Autodesk Inventor part; units mm, degrees
ref_plane "YZ Plane" through (0, 0, 0) normal (1, 0, 0) x (0, 1, 0)
ref_plane "XZ Plane" through (0, 0, 0) normal (0, 1, 0) x (-1, 0, 0)
ref_plane "XY Plane" through (0, 0, 0) normal (0, 0, 1) x (1, 0, 0)
sketch "Sketch1" plane through (0, 0, 0) normal (0, 1, 0) x (-1, 0, 0)
  line L0 (-55.3, 34) -> (55.3, -34) construction
  line L1 (55.3424, 32) -> (55.3424, 21)
  line L2 (53.3, 10) -> (55.3, 10)
  line L3 (55.3, 10) -> (55.3, -1)
  line L4 (55.3, -1) -> (53.3, -1)
  line L5 (53.3, -1) -> (53.3, -12)
  line L6 (53.3, -12) -> (55.3, -12)
  line L7 (55.3, -12) -> (55.3, -23)
  line L8 (55.3, -23) -> (53.3, -23)
  line L9 (55.3424, 21) -> (55.3424, 32)
  line L10 (55.3, -23) -> (55.3, -12)
  line L11 (55.3, -1) -> (55.3, 10)
  line L12 (-53.3, 0.4465) -> (-53.3, 0.446)
  line L13 (-53.3487, -21) -> (-53.3, -21)
  line L14 (55.3424, 32) -> (37.0424, 32)
  line L15 (37.0424, 32) -> (37.0424, 34)
  line L16 (37.0424, 34) -> (18.7424, 34)
  line L17 (18.7424, 34) -> (18.7424, 32)
  line L18 (18.7424, 32) -> (-1.6, 32)
  line L19 (-1.6, 32) -> (-1.6, 34)
  line L20 (-1.6, 34) -> (-17.9, 34)
  line L21 (-17.9, 34) -> (-17.9, 32)
  line L22 (-17.9, 32) -> (-36.2, 32)
  line L23 (-36.2, 32) -> (-36.2, 34)
  line L24 (37.0424, 34) -> (18.7424, 34)
  line L25 (-1.6, 34) -> (-17.9, 34)
  line L26 (-36.2, 34) -> (-55.3, 34)
  line L27 (2.5632, 10.7554) -> (14.3549, 2.3144)
  line L28 (0.7434, 10.7554) -> (-11.0739, 2.3144)
  line L29 (19.1722, 2.3144) -> (2.5632, 14.178)
  line L30 (0.7434, 14.1963) -> (-15.8912, 2.3144)
  line L31 (-20.6639, 0.446) -> (0.7434, -14.8449)
  line L32 (2.5632, -14.8267) -> (23.9449, 0.446)
  line L33 (23.9895, 2.3144) -> (2.5632, 17.6189)
  line L34 (0.7434, 17.6372) -> (-20.7085, 2.3144)
  line L35 (-25.4812, 0.446) -> (0.7434, -18.2859)
  line L36 (2.5632, -18.2676) -> (28.7623, 0.446)
  line L37 (28.8068, 2.3144) -> (2.5632, 21.0599)
  line L38 (41.2856, 32.5499) -> (41.2856, 32.5817)
  line L39 (54.8971, 24.1408) -> (54.9227, 24.1408)
  line L40 (14.3549, 0.446) -> (14.3549, 0.4779)
  line L41 (0.7434, 21.0782) -> (-25.5258, 2.3144)
  line L42 (-11.0739, 2.3144) -> (-15.8912, 2.3144)
  line L43 (-20.7085, 2.3144) -> (-25.5258, 2.3144)
  line L44 (0.7434, 21.0782) -> (0.7434, 17.6372)
  line L45 (0.7434, 14.1963) -> (0.7434, 10.7554)
  line L46 (2.5632, 10.7554) -> (2.5632, 14.178)
  line L47 (2.5632, 17.6189) -> (2.5632, 21.0599)
  line L48 (14.3549, 2.3144) -> (19.1722, 2.3144)
  line L49 (23.9895, 2.3144) -> (28.8068, 2.3144)
  line L50 (28.7623, 0.446) -> (23.9449, 0.446)
  line L51 (2.5632, -14.8267) -> (2.5632, -18.2676)
  line L52 (0.7434, -18.2859) -> (0.7434, -14.8449)
  line L53 (-25.4812, 0.446) -> (-20.6639, 0.446)
  line L54 (-11.0739, 0.4464) -> (-15.8912, 0.4464)
  line L55 (0.7434, -7.9945) -> (-11.0739, 0.4464)
  line L56 (0.7434, -11.4354) -> (-15.8912, 0.4464)
  line L57 (0.7434, -11.4354) -> (0.7434, -7.9945)
  line L58 (-11.7935, 1.3804) -> (-5.9618, 1.3804)
  line L59 (2.5632, 10.7554) -> (2.5632, 10.7554)
  line L60 (2.5632, -7.9945) -> (2.5632, -11.4171)
  line L61 (14.3549, 0.4464) -> (19.1722, 0.4464)
  line L62 (19.1722, 0.4464) -> (2.5632, -11.4171)
  line L63 (2.5632, -7.9945) -> (14.3549, 0.4464)
  line L64 (19.1722, 0.4464) -> (14.3549, 0.4464)
  line L65 (14.3549, 0.4464) -> (2.5632, -7.9945)
  line L66 (2.5632, -7.9945) -> (2.5632, -11.4171)
  line L67 (2.5632, -11.4171) -> (19.1722, 0.4464)
  line L68 (53.3, 10) -> (53.3, 21)
  line L69 (53.3, 21) -> (55.3424, 21)
  line L70 (53.3, -34.0004) -> (53.3, -34.0004)
  line L71 (53.3, -23) -> (53.3, -32)
  line L72 (34.2, -32.0004) -> (34.2, -32)
  line L73 (55.3, 34) -> (-52.0471, -32) construction
  line L74 (53.3, -32) -> (53.3, -34.0004)
  line L75 (-39, -36.0004) -> (-53.3, -36.0004)
  line L76 (-53.3, -36.0004) -> (-57.3, -36.0004)
  line L77 (-57.3, -36.0004) -> (-57.3, -21.0004)
  line L78 (-57.3, -21.0004) -> (-59.3, -21.0004)
  line L79 (-59.3, -21.0004) -> (-59.3, -9.7058)
  line L80 (-59.3, -9.7058) -> (-57.3, -9.7058)
  line L81 (-57.3, -9.7058) -> (-57.3, 0.4464)
  line L82 (-57.3, 0.4464) -> (-57.3, 1)
  line L83 (-57.3, 1) -> (-59.3, 1)
  line L84 (-59.3, 1) -> (-59.3, 12)
  line L85 (-59.3, 12) -> (-57.3, 12)
  line L86 (-57.3, 12) -> (-57.3, 23)
  line L87 (-57.3, 23) -> (-59.3, 23)
  line L88 (-59.3, 23) -> (-59.3, 34)
  line L89 (-59.3, 34) -> (-55.3, 34)
  line L90 (-53.3, -21) -> (-53.3, -21.0004)
  line L91 (-55.3, 32.0365) -> (-55.3, 32)
  line L92 (-55.3, 32.0365) -> (-55.3, 32)
  line L93 (-39, -36.0004) -> (-38.1942, -36.0004)
  line L94 (53.3, -34.0004) -> (35, -34.0004)
  line L95 (35, -34.0004) -> (35, -36.0004)
  line L96 (35, -36.0004) -> (18.7, -36.0004)
  line L97 (18.7, -36.0004) -> (16.7, -36.0004)
  line L98 (16.7, -36.0004) -> (16.7, -34.0004)
  line L99 (16.7, -34.0004) -> (-1.6, -34.0004)
  line L100 (-1.6, -34.0004) -> (-1.6, -36.0004)
  line L101 (-1.6, -36.0004) -> (-17.9, -36.0004)
  line L102 (-17.9, -36.0004) -> (-19.9, -36.0004)
  line L103 (-19.9, -36.0004) -> (-19.9, -34.0004)
  line L104 (-19.9, -34.0004) -> (-38.2, -34.0004)
  line L105 (-38.2, -34.0004) -> (-38.1942, -36.0004)
  point P0 (0, 0)
  point P1 (-53.3, 20.3166)
  point P2 (-53.3, 1)
  point P3 (-53.3, -10)
  point P4 (-55.3, -18.9529)
  point P5 (-53.3, -32.7703)
  point P6 (-16.7, -32.027)
  point P7 (-21.4801, -32.0004)
  point P8 (-17.9, -36.0004)
  dimension "d30" = 1.868
  dimension "d31" = 0.934
  dimension "d34" = 11
  dimension "d35" = 11
  dimension "d36" = 11
  dimension "d37" = 11
  dimension "d38" = 11
  dimension "d61" = 4
  dimension "d70" = 18.3
  dimension "d72" = 2
  dimension "d73" = 18.3
  dimension "d75" = 2
extrude "Extrusion1" add sketch "Sketch1" along normal blind 2
properties part number "ATAS"
Part model, mm, in its own coordinate system. A direction names the side the tool comes from. Round coordinates to 2 decimals unless told otherwise and drop trailing zeros. Loops run counter-clockwise (first coordinate to the right, second up) from the corner with the lowest first, then second, coordinate; pieces in that order, holes last. Notation, with made-up numbers: (79, -37) -> (111, -37) arc R7 ccw to (111, -31) -> close; hole circle Ø11 at (-32.75, -32.75). An arc over 180 degrees is marked (long way). Use one line per item in the form item = value. Start each with the question number.
Item 1: Band-saw the part on C-C (z = -5.5). List the corners of the cut face in (x, y), plus the area to 3 significant figures.
Item 2: Band-saw the part on D-D (y = 1.5). Give the number of separate pieces and of enclosed holes in the cut face, plus the area to 3 significant figures.
Item 3: Tool access for faces 1 (the flat face through (3, 0, -1)), 2 (the flat face through (12.207, 0.986, 11.828)): list every direction of +Z, -Z, +X, -X, +Y, -Y with a clear straight run to the whole face (end or side of a thin tool).
Item 4: Drop flat-ended pins along their axis: pin 1 Ø0.6 at (y, z) = (1.5, 20) entering from +X; pin 2 Ø1 at (x, y) = (-6.5, 1) entering from -Z; pin 3 Ø1 at (x, y) = (18.5, 1) entering from +Z. Give the stop position or say it passes through.
Item 5: Drill centre lines: line 1 along Z through (x, y) = (-8, 0.45); line 2 along X through (y, z) = (1.9, -1.5); line 3 along Z through (x, y) = (14.5, 0.35). Where is each one in solid material? Low to high.
Item 6: Band-saw the part on A-A (z = -13.5). List the corners of the cut face in (x, y).
Item 7: Band-saw the part on B-B (x = -21). List the corners of the cut face in (y, z).
Item 8: Two-plate mould, pull along Z, no slides. Class faces 3 (the flat face through (7.457, 0.986, 8.339)), 4 (the flat face through (-10.984, 0.986, -5.402)), 5 (the flat face through (3, 2, -1)): released by +Z, released by -Z, zero draft, split by the parting line, or undercut.
Data:
q1.outline = (-53.3, 0) -> (-20.44, 0) -> (-20.44, 2) -> (-53.3, 2) -> close; (-15.62, 0) -> (-10.85, 0) -> (-10.85, 2) -> (-15.62, 2) -> close; (-6.05, 0) -> (2.75, 0) -> (2.75, 2) -> (-6.05, 2) -> close; (7.57, 0) -> (12.34, 0) -> (12.34, 2) -> (7.57, 2) -> close; (17.16, 0) -> (57.3, 0) -> (57.3, 2) -> (17.16, 2) -> close
q1.area = 183 mm^2
q2.separate_pieces = 1
q2.enclosed_holes = 8
q2.area = 7,130 mm^2
q3.face_1 = +Z, -Z, +X, -X, -Y
q3.face_2 = +Y, -Y
q4.pin_1 = 57.3
q4.pin_2 = -34
q4.pin_3 = 32
q5.line_1 = -34 to -14.38, -10.94 to -7.53, -4.1 to 6.86, 10.29 to 13.74, 17.18 to 32
q5.line_2 = -53.3 to -26.04, -21.22 to -16.45, -11.64 to 8.35, 13.17 to 17.94, 22.76 to 57.3
q5.line_3 = -36 to -7.4, -3.96 to -0.55, 0.45 to 2.31, 3.31 to 6.75, 10.19 to 34
q6.outline = (-55.3, 0) -> (-9.24, 0) -> (-9.24, 2) -> (-55.3, 2) -> close; (-4.42, 0) -> (1.14, 0) -> (1.14, 2) -> (-4.42, 2) -> close; (5.96, 0) -> (59.3, 0) -> (59.3, 2) -> (5.96, 2) -> close
q7.outline = (0, -36) -> (2, -36) -> (2, -5.1) -> (0, -5.1) -> close; (0, -1.66) -> (2, -1.66) -> (2, 4.45) -> (0, 4.45) -> close; (0, 7.89) -> (2, 7.89) -> (2, 34) -> (0, 34) -> close
q8.face_3 = undercut
q8.face_4 = undercut
q8.face_5 = zero draft
